The model under review builds one solid part; all positions refer to its coordinate system, in mm. A direction names the side the tool comes from. Round coordinates to 2 decimals unless told otherwise and drop trailing zeros. Loops run counter-clockwise (first coordinate to the right, second up) from the corner with the lowest first, then second, coordinate; pieces in that order, holes last. Notation, with made-up numbers: M 1.25,86.5 L 48.25,86.5 A23 ccw 48.25,105.5 Z; hole C 62,66.25 d2. An arc over 180 degrees is marked long. Return JSON: item names as keys, results as strings. Group by question number.
Q1. Consider section A-A (x = 0). State the section outline as (y, z) points.
Q2. To check wall thickness, follow line 1 along Y through (x, z) = (0, 36.4); line 2 along Z through (x, y) = (3.5, 27.5); line 3 along Y through (x, z) = (-12.5, 13.5). State the ranges of each line that lie inside material, in increasing order.
Q3. Clearance check with flat-ended pins moving along their axes: pin 1 Ø1.5 at (x, z) = (2.5, 29) entering from +Y; pin 2 Ø1 at (x, z) = (-6, 22.5) entering from -Y; pin 3 Ø21 at (x, y) = (13, 9.5) entering from -Z; pin 4 Ø6 at (y, z) = (10.5, 11.5) entering from -X. State where each tip first meets the part, or that it passes through.
Q4. Draft analysis for pull direction Y (two halves, no side actions). For faces 4 (the face through (10.382, -19.961, 18.241)), 5 (the face through (23.846, 7.509, 36.507)), 6 (the face through (-4.88, 37.18, 18.24)), 7 (the face through (-31, 17, 37)), state which applies: pulls with the +Y half, pulls with the -Y half, needs draft (parallel to the pull), parting line crosses it, or undercut.
Q5. For faces 1 (the face through (-22.34, 3.82, 37)), 2 (the face through (23.846, 7.509, 0.493)), 3 (the face through (-24, 8, 36)), list the 3-axis set-ups (+Z, -Z, +X, -X, +Y, -Y) from which the entire face can be reached by the end or side of a thin tool; tool diameter is ignored.
Q6. Consider section D-D (y = -27). State the section outline as (x, z) points, and give its area (3 significant figures).
Q7. Consider section C-C (z = 14). State the section outline as (x, y) points.
from build123d import *

# Parameters (mm, degrees)
SZKIC1_R                    = 37.5
SZKIC1_R_2                  = 22.5
DODANIE_WYCI_GNI_CIE1_DEPTH = 37
SZKIC2_R                    = 35
SZKIC2_R_2                  = 25
WYTNIJ_WYCI_GNI_CIE1_DEPTH  = 1


with BuildPart() as part:
    # Szkic1 → Dodanie-wyciągnięcie1 (new body)
    with BuildSketch(Plane.XY):
        Circle(SZKIC1_R)
        Circle(SZKIC1_R_2, mode=Mode.SUBTRACT)
    extrude(amount=DODANIE_WYCI_GNI_CIE1_DEPTH)

    # Szkic2 → Wytnij-wyciągnięcie1 (cut)
    with BuildSketch(Plane.XY.offset(37)):
        Circle(SZKIC2_R)
        Circle(SZKIC2_R_2, mode=Mode.SUBTRACT)
    wytnij_wyci_gni_cie1 = extrude(amount=-WYTNIJ_WYCI_GNI_CIE1_DEPTH, mode=Mode.SUBTRACT)

    # Lustro1: Wytnij-wyciągnięcie1 across plane
    add(wytnij_wyci_gni_cie1.mirror(Plane.XY.offset(18.5)), mode=Mode.SUBTRACT)


solid = part.part
Values:
{
 "1": {"outline": "M -37.5,0 L -35,0 L -35,1 L -25,1 L -25,0 L -22.5,0 L -22.5,37 L -25,37 L -25,36 L -35,36 L -35,37 L -37.5,37 Z; M 22.5,0 L 25,0 L 25,1 L 35,1 L 35,0 L 37.5,0 L 37.5,37 L 35,37 L 35,36 L 25,36 L 25,37 L 22.5,37 Z"},
 "2": {"line 1": "y = -37.5 to -35, -25 to -22.5, 22.5 to 25, 35 to 37.5", "line 2": "z = 1 to 36", "line 3": "y = -35.36 to -18.71, 18.71 to 35.36"},
 "3": {"pin 1": "stops at y = 37.46", "pin 2": "stops at y = -37.09", "pin 3": "stops at z = 0", "pin 4": "stops at x = -36.74"},
 "4": {"face 4": "undercut", "face 5": "undercut", "face 6": "parting line crosses it", "face 7": "needs draft"},
 "5": {"face 1": "+Z, +X, -X, +Y, -Y", "face 2": "-Z", "face 3": "+Z"},
 "6": {"outline": "M -26.02,0 L -22.27,0 L -22.27,1 L 22.27,1 L 22.27,0 L 26.02,0 L 26.02,37 L 22.27,37 L 22.27,36 L -22.27,36 L -22.27,37 L -26.02,37 Z", "area": "1,840 mm2"},
 "7": {"outline": "C 0,0 d75; hole C 0,0 d45"}
}
